```python
from build123d import *

# Parameters (mm, degrees)
SKETCH1_W           = 26
SKETCH1_H           = 17.6
SKETCH1_R           = 1.75
BOSS_EXTRUDE1_DEPTH = 4.5
SKETCH2_W           = 12
SKETCH2_H           = 4.2
BOSS_EXTRUDE2_DEPTH = 3.5
SKETCH3_W           = 9
SKETCH3_H           = 1.5
CUT_EXTRUDE1_DEPTH  = 1.5
SKETCH4_W           = 20
SKETCH4_H           = 7.5
BOSS_EXTRUDE3_DEPTH = 6.75
SKETCH5_W           = 0.5
SKETCH5_H           = 0.5
BOSS_EXTRUDE4_DEPTH = 8


with BuildPart() as part:
    # Sketch1 → Boss-Extrude1 (new body)
    with BuildSketch(Plane(origin=(0, 0, 0), x_dir=(1, 0, 0), z_dir=(0, 1, 0))):
        Rectangle(SKETCH1_W, SKETCH1_H)
        with Locations((10, -5.3)):
            Circle(SKETCH1_R, mode=Mode.SUBTRACT)
        with Locations((-10, -5.3)):
            Circle(SKETCH1_R, mode=Mode.SUBTRACT)
    extrude(amount=BOSS_EXTRUDE1_DEPTH)

    # Sketch2 → Boss-Extrude2 (add)
    with BuildSketch(Plane(origin=(0, 4.5, 0), x_dir=(1, 0, 0), z_dir=(0, 1, 0))):
        with Locations((0, -6.7)):
            Rectangle(SKETCH2_W, SKETCH2_H)
    extrude(amount=BOSS_EXTRUDE2_DEPTH)

    # Sketch3 → Cut-Extrude1 (cut)
    with BuildSketch(Plane.XY.offset(8.8)):
        with Locations((0, 6.25)):
            Rectangle(SKETCH3_W, SKETCH3_H)
    extrude(amount=-CUT_EXTRUDE1_DEPTH, mode=Mode.SUBTRACT)

    # Sketch4 → Boss-Extrude3 (add)
    with BuildSketch(Plane(origin=(0, 4.5, 0), x_dir=(1, 0, 0), z_dir=(0, 1, 0))):
        with Locations((0, 5.05)):
            Rectangle(SKETCH4_W, SKETCH4_H)
    extrude(amount=BOSS_EXTRUDE3_DEPTH)

    # Sketch5 → Boss-Extrude4 (add)
    with BuildSketch(Plane(origin=(0, 0, -8.8), x_dir=(-1, 0, 0), z_dir=(0, 0, -1))):
        with Locations((3.25, 7.875)):
            Rectangle(SKETCH5_W, SKETCH5_H)
        with Locations((1.25, 7.875)):
            Rectangle(SKETCH5_W, SKETCH5_H)
        with Locations((5.25, 7.875)):
            Rectangle(SKETCH5_W, SKETCH5_H)
        with Locations((7.25, 7.875)):
            Rectangle(SKETCH5_W, SKETCH5_H)
        with Locations((-7.25, 7.875)):
            Rectangle(SKETCH5_W, SKETCH5_H)
        with Locations((-5.25, 7.875)):
            Rectangle(SKETCH5_W, SKETCH5_H)
        with Locations((-3.25, 7.875)):
            Rectangle(SKETCH5_W, SKETCH5_H)
        with Locations((-1.25, 7.875)):
            Rectangle(SKETCH5_W, SKETCH5_H)
        with Locations((-3.25, 9.875)):
            Rectangle(SKETCH5_W, SKETCH5_H)
        with Locations((-1.25, 9.875)):
            Rectangle(SKETCH5_W, SKETCH5_H)
        with Locations((-5.25, 9.875)):
            Rectangle(SKETCH5_W, SKETCH5_H)
        with Locations((-7.25, 9.875)):
            Rectangle(SKETCH5_W, SKETCH5_H)
        with Locations((7.25, 9.875)):
            Rectangle(SKETCH5_W, SKETCH5_H)
        with Locations((5.25, 9.875)):
            Rectangle(SKETCH5_W, SKETCH5_H)
        with Locations((3.25, 9.875)):
            Rectangle(SKETCH5_W, SKETCH5_H)
        with Locations((1.25, 9.875)):
            Rectangle(SKETCH5_W, SKETCH5_H)
        with Locations((-3.25, 5.875)):
            Rectangle(SKETCH5_W, SKETCH5_H)
        with Locations((-1.25, 5.875)):
            Rectangle(SKETCH5_W, SKETCH5_H)
        with Locations((-5.25, 5.875)):
            Rectangle(SKETCH5_W, SKETCH5_H)
        with Locations((-7.25, 5.875)):
            Rectangle(SKETCH5_W, SKETCH5_H)
        with Locations((7.25, 5.875)):
            Rectangle(SKETCH5_W, SKETCH5_H)
        with Locations((5.25, 5.875)):
            Rectangle(SKETCH5_W, SKETCH5_H)
        with Locations((3.25, 5.875)):
            Rectangle(SKETCH5_W, SKETCH5_H)
        with Locations((1.25, 5.875)):
            Rectangle(SKETCH5_W, SKETCH5_H)
    extrude(amount=BOSS_EXTRUDE4_DEPTH)


solid = part.part
```
CAD build for the part. Positions are in the model's coordinates, mm. A direction names the side the tool comes from. Coordinates: 2 decimals unless noted, no trailing zeros. Order: outer loops, then holes, each group sorted by start corner. A loop starts at its lowest first (then second) coordinate and runs counter-clockwise, first axis right, second up. Notation, with made-up numbers: (20, 51) - (77, 51) arc R22 ccw to (77, 67) - close; hole circle Ø1 at (86, 44). An arc over 180 degrees is marked (long way). Answer in a Markdown table with one row per item.
1. Drill centre lines: L1, parallel to X at y = 3.3, z = 5.3; L2, parallel to Z at x = -10, y = 2.1; L3, parallel to Z at x = 4, y = 6.5. Where is each one in solid material? Low to high. Write a range as from..to.
Answer:
| item | result |
|---|---|
| L1 | -13..-11.75, -8.25..8.25, 11.75..13 |
| L2 | -8.8..3.55, 7.05..8.8 |
| L3 | -8.8..-1.3, 4.6..7.3 |
2. Slice it at A-A, the plane y = 1.25. List the corners of the cut face in (x, z).
Answer:
| item | result |
|---|---|
| outline | (-13, -8.8) - (13, -8.8) - (13, 8.8) - (-13, 8.8) - close; hole circle Ø3.5 at (-10, 5.3); hole circle Ø3.5 at (10, 5.3) |
3. Slice it at C-C, the plane z = -7.5. List the corners of the cut face in (x, y).
Answer:
| item | result |
|---|---|
| outline | (-13, 0) - (13, 0) - (13, 4.5) - (10, 4.5) - (10, 11.25) - (-10, 11.25) - (-10, 4.5) - (-13, 4.5) - close |
4. 3-axis set-ups, long thin cutter, end or side, ignore diameter. For faces 1 (the face through (4.5, 6, 8)), 2 (the face through (0, 6, 4.6)), 3 (the face through (10, 8, -5)), 4 (the face through (-6, 6, 7)), 5 (the face through (-10, 8, -5)): which of +Z, -Z, +X, -X, +Y, -Y reach the whole face in a straight line?
Answer:
| item | result |
|---|---|
| face 1 | +Z |
| face 2 | +X, -X, +Y |
| face 3 | +Z, -Z, +X, +Y |
| face 4 | +Z, -X, +Y |
| face 5 | +Z, -Z, -X, +Y |
5. Slice it at B-B, the plane z = 5.3. List the corners of the cut face in (x, y), then the cut area to 4 significant figures.
Answer:
| item | result |
|---|---|
| outline | (-13, 0) - (-11.75, 0) - (-11.75, 4.5) - (-13, 4.5) - close; (-8.25, 0) - (8.25, 0) - (8.25, 4.5) - (6, 4.5) - (6, 8) - (-6, 8) - (-6, 4.5) - (-8.25, 4.5) - close; (11.75, 0) - (13, 0) - (13, 4.5) - (11.75, 4.5) - close |
| area | 127.5 mm² |
6. Flat gauge pins, fed straight in: P1, Ø3, axis at x = 1, z = -6.5, coming from the -Y side; P2, Ø2, axis at y = 7, z = -5, coming from the -X side; P3, Ø1, axis at x = 0.5, y = 7, coming from the -Z side; P4, Ø0.6, axis at y = 6, z = -13, coming from the +X side. Where does each tip first touch, or does it go through?
Answer:
| item | result |
|---|---|
| P1 | y = 0 |
| P2 | x = -10 |
| P3 | z = -8.8 |
| P4 | x = 7.5 |
7. Pull direction Y, two halves, no side cores. Call faces 6 (the face through (0, 11.25, -5)), 7 (the face through (-4.5, 6, 8)), 8 (the face through (13, 2, 0)), 9 (the face through (0, 6, 7.3)): +Y half, -Y half, draft (parallel to the pull), parting line (faces both ways), or undercut.
Answer:
| item | result |
|---|---|
| face 6 | +Y half |
| face 7 | undercut |
| face 8 | draft |
| face 9 | undercut |
8. Slice it at D-D, the plane x = 9. List the corners of the cut face in (y, z).
Answer:
| item | result |
|---|---|
| outline | (0, -8.8) - (11.25, -8.8) - (11.25, -1.3) - (4.5, -1.3) - (4.5, 3.86) - (0, 3.86) - close; (0, 6.74) - (4.5, 6.74) - (4.5, 8.8) - (0, 8.8) - close |
